Input: part model. Units: mm. Frame: model coordinates. Face numbers are marked on the shaded views. Give positions to 0.01 mm unless a question says otherwise; leave off trailing zeros. Loops run counter-clockwise (first coordinate to the right, second up) from the corner with the lowest first, then second, coordinate; pieces in that order, holes last.
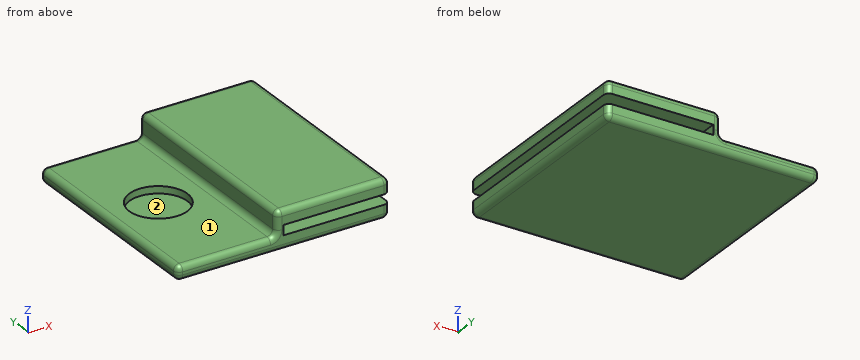
from build123d import *

# Parameters (mm, degrees)
F0_W     = 75
F0_H     = 75
F1_DEPTH = 5
F2_W     = 40
F2_H     = 75
F3_DEPTH = 8.5
F4_W     = 75
F4_H     = 3.5
F5_DEPTH = 37.5
F6_R     = 10.25
F7_DEPTH = 2.5
F8_R     = 2


with BuildPart() as f1:
    # F0 (on Top) → F1 (new body)
    with BuildSketch(Plane.XY):
        Rectangle(F0_W, F0_H)
    extrude(amount=F1_DEPTH)

    # F2 (on face) → F3 (join)
    with BuildSketch(Plane.XY.offset(5)):
        with Locations((17.5, 0)):
            Rectangle(F2_W, F2_H)
    extrude(amount=F3_DEPTH)

    # F4 (on face) → F5 (cut, through all)
    with BuildSketch(Plane.YZ.offset(37.5)):
        with Locations((0, 6.75)):
            Rectangle(F4_W, F4_H)
    extrude(amount=-F5_DEPTH, mode=Mode.SUBTRACT)

    # F6 (on face) → F7 (cut)
    with BuildSketch(Plane.XY.offset(5)):
        with Locations((-20, 0)):
            Circle(F6_R)
    extrude(amount=-F7_DEPTH, mode=Mode.SUBTRACT)

    # F8
    f8_edges = [f1.edges().sort_by_distance(p)[0] for p in [
        (17.5, 37.5, 13.5),
        (-2.5, 0, 13.5),
        (17.5, -37.5, 13.5),
        (37.5, 0, 13.5),
        (-2.5, 37.5, 9.25),
        (-2.5, -37.5, 9.25),
        (-2.5, 0, 5),
        (-37.5, 37.5, 2.5),
        (-37.5, -37.5, 2.5),
        (-37.5, 0, 0),
        (-37.5, 0, 5),
        (0, -37.5, 0),
        (37.5, 0, 0),
        (0, 37.5, 0),
        (37.5, -37.5, 11),
        (37.5, -37.5, 2.5),
        (37.5, 37.5, 11),
        (37.5, 37.5, 2.5),
        (-20, -37.5, 5),
        (-20, 37.5, 5),
    ]]
    fillet(f8_edges, radius=F8_R)


solid = f1.part
(1) Mould query, pull axis X, two halves, no side actions, for the marked faces 1 and 2. Classes: +X half, -X half, draft (parallel to the pull), parting line (faces both ways), or undercut.
Values follow:
face 1: draft
face 2: undercut
(2) Cut plane C-C (x = -20). Return the cut outline in (y, z).
Values follow:
outline: (-37.5, 2) arc R2 ccw to (-35.5, 0) - (35.5, 0) arc R2 ccw to (37.5, 2) - (37.5, 3) arc R2 ccw to (35.5, 5) - (10.25, 5) - (10.25, 2.5) - (-10.25, 2.5) - (-10.25, 5) - (-35.5, 5) arc R2 ccw to (-37.5, 3) - close
(3) Cut plane B-B (y = 0). Return the cut outline in (x, z), and give its area (3 significant figures).
Values follow:
outline: (-37.5, 2) arc R2 ccw to (-35.5, 0) - (35.5, 0) arc R2 ccw to (37.5, 2) - (37.5, 5) - (0, 5) - (0, 8.5) - (37.5, 8.5) - (37.5, 11.5) arc R2 ccw to (35.5, 13.5) - (-0.5, 13.5) arc R2 ccw to (-2.5, 11.5) - (-2.5, 7) arc R2 cw to (-4.5, 5) - (-9.75, 5) - (-9.75, 2.5) - (-30.25, 2.5) - (-30.25, 5) - (-35.5, 5) arc R2 ccw to (-37.5, 3) - close
area: 529 mm2
(4) Ray query, probe 1 along Z at (x, y) = (16, 26.5); probe 2 along X at (y, z) = (-2, 8.75); probe 3 along Y at (x, z) = (-20, 3.65). Return the intervals inside material, ascending.
Values follow:
probe 1: z = 0 to 5, 8.5 to 13.5
probe 2: x = -2.5 to 37.5
probe 3: y = -37.39 to -10.25, 10.25 to 37.39
(5) Pin query (flat end, axial travel): pin 1 Ø1.5 at (x, z) = (16, 5.5) entering from +Y; pin 2 Ø16.5 at (x, y) = (-16.5, -5) entering from +Z; pin 3 Ø1.5 at (y, z) = (30, 6.5) entering from -X; pin 4 Ø2 at (y, z) = (10, 8.5) entering from -X. Return the tip coordinate at first contact, or that it passes through.
Values follow:
pin 1: stops at y = 37.5
pin 2: stops at z = 5
pin 3: stops at x = -2.94
pin 4: stops at x = -2.5
(6) Cut plane A-A (x = 12.5). Return the cut outline in (y, z), and give its area (3 significant figures).
Values follow:
outline: (-37.5, 2) arc R2 ccw to (-35.5, 0) - (35.5, 0) arc R2 ccw to (37.5, 2) - (37.5, 5) - (-37.5, 5) - close; (-37.5, 8.5) - (37.5, 8.5) - (37.5, 11.5) arc R2 ccw to (35.5, 13.5) - (-35.5, 13.5) arc R2 ccw to (-37.5, 11.5) - close
area: 747 mm2
(7) Cut plane D-D (y = 15). Return the cut outline in (x, z), and give its area (3 significant figures).
Values follow:
outline: (-37.5, 2) arc R2 ccw to (-35.5, 0) - (35.5, 0) arc R2 ccw to (37.5, 2) - (37.5, 5) - (0, 5) - (0, 8.5) - (37.5, 8.5) - (37.5, 11.5) arc R2 ccw to (35.5, 13.5) - (-0.5, 13.5) arc R2 ccw to (-2.5, 11.5) - (-2.5, 7) arc R2 cw to (-4.5, 5) - (-35.5, 5) arc R2 ccw to (-37.5, 3) - close
area: 580 mm2
